Can you work these out from the model? Positions are in its coordinate system, mm. A direction names the side the tool comes from. Coordinates: 2 decimals unless noted, no trailing zeros. Order: outer loops, then holes, each group sorted by start corner. A loop starts at its lowest first (then second) coordinate and runs counter-clockwise, first axis right, second up. Notation, with made-up numbers: M 51.5,26.25 L 91.5,26.25 A24 cw 91.5,59.25 Z; hole C 63.25,-15 d11. An arc over 180 degrees is marked long. Answer as CSV lines item,"result". Start each with the question number.
1. If we section it at C-C (x = 12.7): List the corners of the cut face in (y, z) for me.
2. I need wall thicknesses on line 1 along Y through (x, z) = (12.7, 5.25); line 2 along X through (y, z) = (31.5, 9.25); line 3 along Y through (x, z) = (63.5, 3.4). Which ranges of each line are inside material? Lowest first, please. Write a range as from..to.
3. Will these pins go through, and if not, where does the flat tip stop? pin 1 (9.5 mm diameter, centred on x = 63.5, y = 31.75, fed in from +Z); pin 2 (5.5 mm diameter, centred on x = 11.5, y = 10.5, fed in from -Z).
4. On a 3-axis mill with a long thin cutter (end or side, diameter ignored), from which of +Z, -Z, +X, -X, +Y, -Y can I reach the whole of each face in a straight line? I mean faces 1 (the face through (12.235, 13.066, 9.569)), 2 (the face through (59.4, 35.5, 9.2)), 3 (the face through (9, 10, 6.35)). Say none if no direction works.
5. If we section it at B-B (x = 31.75): List the corners of the cut face in (y, z) for me.
6. If we section it at D-D (y = 7): List the corners of the cut face in (x, z) for me.
7. If we section it at A-A (y = 31.75): List the corners of the cut face in (x, z) for me, plus the area to 3 significant figures.
8. If we mould it in two halves opening along X, with no side actions, what happens to faces 4 (the face through (95.25, 31, 6)), 5 (the face through (47, 63.5, 6)), 6 (the face through (14.35, 50.81, 9.57))? For each: released by +X, released by -X, zero draft, split by the parting line, or undercut.
```python
from build123d import *

# Parameters (mm, degrees)
SKETCH1_W                                        = 95.25
SKETCH1_H                                        = 63.5
BOSS_EXTRUDE1_DEPTH                              = 12.7
CBORE_FOR_1_4_SOCKET_HEAD_CAP_SCREW1_D           = 7.14248
CBORE_FOR_1_4_SOCKET_HEAD_CAP_SCREW1_CBORE_D     = 11.1125
CBORE_FOR_1_4_SOCKET_HEAD_CAP_SCREW1_CBORE_DEPTH = 6.35
CBORE_FOR_1_4_SOCKET_HEAD_CAP_SCREW2_D           = 7.14248
CBORE_FOR_1_4_SOCKET_HEAD_CAP_SCREW2_CBORE_D     = 11.1125
CBORE_FOR_1_4_SOCKET_HEAD_CAP_SCREW2_CBORE_DEPTH = 7.112


with BuildPart() as part:
    # Sketch1 → Boss-Extrude1 (new body)
    with BuildSketch(Plane.XY):
        with Locations((47.625, 31.75)):
            Rectangle(SKETCH1_W, SKETCH1_H)
    extrude(amount=BOSS_EXTRUDE1_DEPTH)

    # CBORE for 1/4 Socket Head Cap Screw1 (through all)
    with Locations(Plane(origin=(0, 0, 0), x_dir=(-1, 0, 0), z_dir=(0, 0, -1))):
        with Locations((-12.7, 53.975), (-12.7, 9.525)):
            CounterBoreHole(CBORE_FOR_1_4_SOCKET_HEAD_CAP_SCREW1_D / 2, CBORE_FOR_1_4_SOCKET_HEAD_CAP_SCREW1_CBORE_D / 2, CBORE_FOR_1_4_SOCKET_HEAD_CAP_SCREW1_CBORE_DEPTH)

    # CBORE for 1/4 Socket Head Cap Screw2 (through all)
    with Locations(Plane.XY.offset(12.7)):
        with Locations((31.75, 31.75), (63.5, 31.75)):
            CounterBoreHole(CBORE_FOR_1_4_SOCKET_HEAD_CAP_SCREW2_D / 2, CBORE_FOR_1_4_SOCKET_HEAD_CAP_SCREW2_CBORE_D / 2, CBORE_FOR_1_4_SOCKET_HEAD_CAP_SCREW2_CBORE_DEPTH)


solid = part.part
```
Solved:
1,outline,"M 0,0 L 3.97,0 L 3.97,6.35 L 5.95,6.35 L 5.95,12.7 L 0,12.7 Z; M 13.1,6.35 L 15.08,6.35 L 15.08,0 L 48.42,0 L 48.42,6.35 L 50.4,6.35 L 50.4,12.7 L 13.1,12.7 Z; M 57.55,6.35 L 59.53,6.35 L 59.53,0 L 63.5,0 L 63.5,12.7 L 57.55,12.7 Z"
2,line 1,"0..3.97, 15.08..48.42, 59.53..63.5"
2,line 2,"0..26.2, 37.3..57.95, 69.05..95.25"
2,line 3,"0..28.18, 35.32..63.5"
3,pin 1,"z = 5.59"
3,pin 2,"z = 6.35"
4,face 1,"+Z, -Z"
4,face 2,"+Z"
4,face 3,"-Z"
5,outline,"M 0,0 L 28.18,0 L 28.18,5.59 L 26.19,5.59 L 26.19,12.7 L 0,12.7 Z; M 35.32,0 L 63.5,0 L 63.5,12.7 L 37.31,12.7 L 37.31,5.59 L 35.32,5.59 Z"
6,outline,"M 0,0 L 7.75,0 L 7.75,6.35 L 10.17,6.35 L 10.17,12.7 L 0,12.7 Z; M 15.23,6.35 L 17.65,6.35 L 17.65,0 L 95.25,0 L 95.25,12.7 L 15.23,12.7 Z"
7,outline,"M 0,0 L 28.18,0 L 28.18,5.59 L 26.19,5.59 L 26.19,12.7 L 0,12.7 Z; M 35.32,0 L 59.93,0 L 59.93,5.59 L 57.94,5.59 L 57.94,12.7 L 37.31,12.7 L 37.31,5.59 L 35.32,5.59 Z; M 67.07,0 L 95.25,0 L 95.25,12.7 L 69.06,12.7 L 69.06,5.59 L 67.07,5.59 Z"
7,area,"972 mm²"
8,face 4,"released by +X"
8,face 5,"zero draft"
8,face 6,"undercut"
